Work out the finished part from the listing and answer in its coordinate system (mm). Face numbers are marked on the shaded views. A direction names the side the tool comes from. Give positions to 0.01 mm unless a question says otherwise; leave off trailing zeros. Loops run counter-clockwise (first coordinate to the right, second up) from the corner with the lowest first, then second, coordinate; pieces in that order, holes last. Notation, with made-up numbers: M 50,62 L 96,62 A13 cw 96,86 Z; hole C -31.5,-15 d8. An arc over 180 degrees is marked long. Use a Markdown table: item, result.
```python
from build123d import *

# Parameters (mm, degrees)
F2_DEPTH  = 6
F4_DEPTH  = 3
F5_DEPTH  = 6.5
F7_DEPTH  = 1.5
F8_R      = 0.99999
F10_DEPTH = 1


# Not quite as in the source:
# - a fillet or chamfer is up to 0.001 mm smaller than in the source, because OpenCascade refuses the exact size


with BuildPart() as f2:
    # F1 (on offset) → F2 (new body)
    with BuildSketch(Plane.XY.offset(4)):
        Polygon((20, 0), (0, 0), (0, 20), (-2.5, 20), (-2.5, -2.5), (20, -2.5), align=None)
    extrude(amount=F2_DEPTH)



with BuildPart() as f4:
    # F3 (on Top) → F4 (new body)
    with BuildSketch(Plane.XY):
        Polygon((16.591883092, 13.7634559673), (16.591883092, 9.5208152802), (4.5710678119, -2.5), (8.75, -2.5), (22.9713253162, 11.5625), (17.2989898732, 17.2989898732), (15.1776695297, 15.1776695297), align=None)
        Polygon((22.9713253162, 11.5625), (8.75, -2.5), (20, -2.5), (20.0004931539, 0), align=None)
        Polygon((13.7634559673, 16.591883092), (15.1776695297, 15.1776695297), (17.2989898732, 17.2989898732), (11.5625, 22.9713253162), (-2.5, 8.75), (-2.5, 4.5710678119), (9.5208152802, 16.591883092), align=None)
        Polygon((-2.5, 8.75), (11.5625, 22.9713253162), (0, 19.9992582202), (-2.5, 20), align=None)
    extrude(amount=-F4_DEPTH)


with BuildPart() as f2_1:
    add(f2.part)

    add(f4.part)  # F5 merges F4
    # F1 (on offset) → F5 (join)
    with BuildSketch(Plane.XY.offset(4)):
        Polygon((20, 0), (0, 0), (0, 20), (-2.5, 20), (-2.5, -2.5), (20, -2.5), align=None)
    extrude(amount=-F5_DEPTH)

    # F6 (on face) → F7 (join)
    with BuildSketch(Plane(origin=(15.1776695297, 15.1776695297, 0), x_dir=(0.7071067812, -0.7071067812, 0), z_dir=(-0.7071067812, -0.7071067812, 0))):
        with BuildLine():
            Line((-1, -3), (1, -3))
            ThreePointArc((1, -3), (0, -2), (-1, -3))
        make_face()
    extrude(amount=F7_DEPTH)

    # F8 (radius 1 in the source; OpenCascade refuses exactly that, so slightly less here)
    f8_edges = [f2_1.edges().sort_by_distance(p)[0] for p in [
        (14.117009, 14.117009, -2),
    ]]
    fillet(f8_edges, radius=F8_R)

    # F9 (on face) → F10 (join)
    with BuildSketch(Plane.XY.offset(10)):
        Polygon((4, 20), (-2.5, 20), (-2.5, -2.5), (20, -2.5), (20, 4), (4, 4), align=None)
    extrude(amount=-F10_DEPTH)


solid = f2_1.part
```
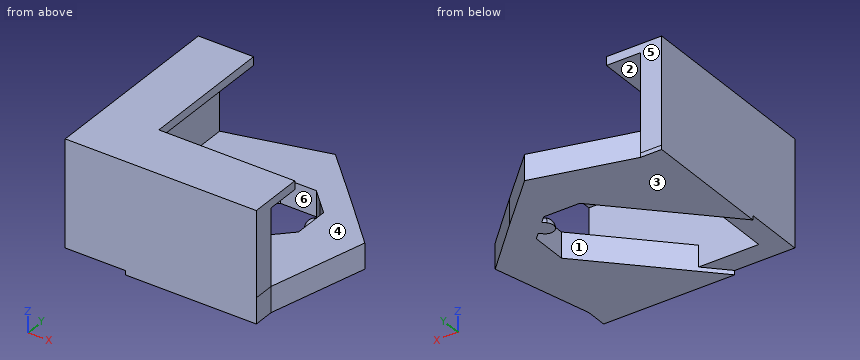
(1) A cutting plane is placed at B-B (x = 5). Write down the section's boundary in (y, z).
Entries:
| item | result |
|---|---|
| outline | M -2.5,-3 L -2.07,-3 L -2.07,-2.5 L 0,-2.5 L 0,9 L 4,9 L 4,10 L -2.5,10 Z; M 12.07,-3 L 21.28,-3 L 21.28,0 L 12.07,0 Z |
(2) A cutting plane is placed at C-C (y = 11). Write down the section's boundary in (x, z).
Entries:
| item | result |
|---|---|
| outline | M -2.5,-3 L 3.93,-3 L 3.93,0 L 0,0 L 0,9 L 4,9 L 4,10 L -2.5,10 Z; M 16.59,-3 L 22.83,-3 L 22.83,0 L 16.59,0 Z |
(3) Which of the six approach directions +Z, -Z, +X, -X, +Y, -Y give full straight-line access (tool end or side, diameter ignored) to the marked faces 4, 5 and 6?
Entries:
| item | result |
|---|---|
| face 4 | +X, +Y |
| face 5 | +Z, -X, +Y |
| face 6 | +Z, -Z |
(4) A cutting plane is placed at D-D (x = 18.75). Write down the section's boundary in (y, z), and give its area (3 significant figures).
Entries:
| item | result |
|---|---|
| outline | M -2.5,-3 L 15.83,-3 L 15.83,0 L 0,0 L 0,9 L 4,9 L 4,10 L -2.5,10 Z |
| area | 84.0 mm² |
(5) Given P1, Ø3.5, axis at x = 6, z = 5.5, coming from the +Y side; P2, Ø4, axis at x = 16, y = 14.5, coming from the +Z side; P3, Ø0.8, axis at y = 14, z = 9.5, coming from the +X side, each flat-ended and moving along its own axis, determine where each tip first touches the part or whether it passes through.
Entries:
| item | result |
|---|---|
| P1 | stops at y = 0 |
| P2 | stops at z = 0 |
| P3 | stops at x = 4 |
(6) The mould has two halves that part along Z. Classify the marked faces 1, 2 and 3: released by +Z, released by -Z, zero draft, split by the parting line, or undercut.
Entries:
| item | result |
|---|---|
| face 1 | zero draft |
| face 2 | undercut |
| face 3 | released by -Z |
(7) Consider probe 1 along Z at (x, y) = (17.75, 3.25); probe 2 along X at (y, z) = (5.5, 5). Determine where each line is inside the solid, lowest interval first. Write a range as [from, to].
Entries:
| item | result |
|---|---|
| probe 1 | z = [-3, 0], [9, 10] |
| probe 2 | x = [-2.5, 0] |
